Read the model definition and answer for the solid it produces. Units are mm, in the model's axes. Round coordinates to 2 decimals unless told otherwise and drop trailing zeros. Order: outer loops, then holes, each group sorted by start corner. A loop starts at its lowest first (then second) coordinate and runs counter-clockwise, first axis right, second up. Notation, with made-up numbers: (34, 37.5) -> (80, 37.5) arc R6 cw to (80, 43.5) -> close; hole circle Ø7 at (-23, 26.25). An arc over 180 degrees is marked (long way). Answer as a JSON object with one key per item and string values. Group by question number.
Item 1: Section A-A, the plane z = -97 is taken. Write down the section's boundary in (x, y), plus the area to 3 significant figures.
Item 2: Consider probe 1 along Z at (x, y) = (37.5, 192); probe 2 along Z at (x, y) = (107, 77); probe 3 along Y at (x, z) = (52, -43). Determine where each line is inside the solid, lowest interval first. Write a range as from..to.
Item 3: Given P1, Ø10, axis at x = 96, z = -154, coming from the -Y side; P2, Ø10, axis at x = 42.5, y = 77.5, coming from the -Z side; P3, Ø3, axis at x = 44, y = 302, coming from the +Z side, each flat-ended and moving along its own axis, determine where each tip first touches the part or whether it passes through.
Item 4: The mould has two halves that part along Z. Classify faces 1 (the flat face through (0, 343, 91)), 2 (the flat face through (78.88, 322.594, -38.801)), 3 (the flat face through (78.88, 352.375, -44.693)): pulls with the +Z half, pulls with the -Z half, needs draft (parallel to the pull), parting line crosses it, or undercut.
Autodesk Inventor part; units mm, degrees
ref_plane "YZ Plane" through (0, 0, 0) normal (1, 0, 0) x (0, 1, 0)
ref_plane "XY Plane" through (0, 0, 0) normal (0, 0, 1) x (1, 0, 0)
sketch "Sketch2" plane through (0, 0, 0) normal (1, 0, 0) x (0, 1, 0)
  line L0 (0, 380) -> (0, 410)
  line L1 (0, -230) -> (0, -200)
  line L2 (0, 0) -> (0, 132.8644)
  line L3 (295.6158, -112.924) -> (350.339, 37.4268)
  line L4 (379.3536, 29.4296) -> (324.6304, -120.9212)
  ellipse E0 centre (0, 0) end of major axis (358.1699, 0) minor radius 200 (0, -200) -> (295.6158, -112.924) ccw
  ellipse E1 centre (0, 0) end of major axis (352.0508, 0) minor radius 380 (350.339, 37.4268) -> (0, 380) ccw
  ellipse E2 centre (0, 0) end of major axis (381.6296, 0) minor radius 230 (0, -230) -> (324.6304, -120.9212) ccw
  ellipse E3 centre (0, 0) end of major axis (380.3347, 0) minor radius 410 (379.3536, 29.4296) -> (0, 410) ccw
  point P0 (0, 0)
  dimension "d10" = 30
  dimension "d11" = 30
  dimension "d12" = 0
  dimension "d16" = 380
  dimension "d17" = 200
  dimension "d25" = 20
  dimension "d26" = 160
  dimension "d27" = 30
  dimension "d28" = 160
extrude "Extrusion1" add sketch "Sketch2" along normal blind 160
sketch "Sketch3" plane through (0, 0, 0) normal (-1, 0, 0) x (0, 0, 1)
  line L0 (171.5389, -307.9404) -> (-54.4979, 313.0907)
  line L1 (-120.9212, 324.6304) -> (29.4296, 379.3536)
  line L2 (-111.428, -307.9404) -> (360.7046, -307.9404)
  line L3 (76.7879, 236.8347) -> (76.7879, -307.9404)
  point P0 (0, 0)
  dimension "d31" = 94.751
sketch "Sketch4" plane through (0, 0, 380) normal (0, -1, 0) x (1, 0, 0)
  line L0 (160, 30) -> (160, 0)
  line L1 (160, -610) -> (160, -500.9212)
  line L2 (160, 30) -> (160, -610)
  line L3 (160, 0) -> (160, -342.5732)
  ellipse E0 centre (160, -290) end of major axis (390, -290) minor radius 320 (160, -610) -> (160, 30) ccw
  line L4 (0, 30) -> (160, 30)
  line L5 (0, 0) -> (160, 0)
  ellipse E1 centre (160, -290) end of major axis (360, -290) minor radius 290 (160, -580) -> (160, 0) ccw
  point P0 (0, -380)
  dimension "d33" = 200
  dimension "d34" = 230
  dimension "d32" = 320
ref_plane "Work Plane3" through (0, 0, 90) normal (0, 0, -1) x (-1, 0, 0)
ref_plane "Work Plane1" through (0, 0, -230) normal (0, 0, -1) x (-1, 0, 0)
ref_plane "Work Plane2" through (0, 0, 410) normal (0, 0, 1) x (1, 0, 0)
sketch "Sketch6" plane through (0, 0, 90) normal (0, 0, -1) x (-1, 0, 0)
  line L0 (-160, 371.0583) -> (0, 371.0583)
  line L1 (0, 371.0583) -> (0, 342.0343)
  line L2 (0, 342.0343) -> (-160, 342.0343)
  line L3 (-160, 342.0343) -> (-160, 371.0583)
  ellipse E0 centre (-160, -10) end of major axis (-390, -10) minor radius 381.0583 (-160, 371.0583) -> (-390, -10) ccw
  line L4 (-160, 0) -> (-160, 350.339)
  line L5 (-160, 342.0343) -> (-160, 371.0583)
  line L6 (-360, -10) -> (-390, -10)
  ellipse E1 centre (-160, -10) end of major axis (-360, -10) minor radius 352.0343 (-160, 342.0343) -> (-360, -10) ccw
  ellipse E2 centre (-160, -10) end of major axis (-403.0676, -10) minor radius 410.7244 (-34.7861, 342.0343) -> (-69.2995, 371.0583) ccw
  line L7 (0, 0) -> (-160, 0)
  point P0 (-160, 324.6304)
  dimension "d62" = 200
  dimension "d63" = 230
  dimension "d58" = 30
  dimension "d59" = 0
  dimension "d60" = 10
  dimension "d61" = 0
sketch "Sketch7" plane through (0, 0, 90) normal (0, 0, -1) x (-1, 0, 0)
  line L0 (0, 0) -> (-160, 0)
  ellipse E0 centre (-160, 0) end of major axis (-160, 365) minor radius 215 (-160, 365) -> (-375, 0) ccw
  line L1 (-160, 0) -> (-160, 350.339)
  line L2 (-375, 0) -> (-160, 0)
  line L3 (-160, 0) -> (-160, 365)
  line L4 (-160, 324.6304) -> (-160, 379.3536)
  dimension "d40" = 215
  dimension "d41" = 365
ref_plane "Work Plane4" through (210, 0, 0) normal (1, 0, 0) x (0, 0, -1)
sketch "Sketch10" plane through (160, 0, 0) normal (1, 0, 0) x (0, 0, -1)
  line L0 (120.9212, 324.6304) -> (-29.4296, 379.3536)
  ellipse E0 centre (0, 0) end of major axis (-410, 0) minor radius 380.3347 (-29.4296, 379.3536) -> (-410, 0) ccw
  line L1 (-410, 0) -> (-380, 0)
  ellipse E1 centre (0, 0) end of major axis (-380, 0) minor radius 352.0508 (-37.4268, 350.339) -> (-380, 0) ccw
  line L2 (-37.4268, 350.339) -> (112.924, 295.6158)
  ellipse E2 centre (0, 0) end of major axis (0, -358.1699) minor radius 200 (200, 0) -> (112.924, 295.6158) ccw
  line L3 (200, 0) -> (230, 0)
  ellipse E3 centre (0, 0) end of major axis (0, 381.6296) minor radius 230 (230, 0) -> (120.9212, 324.6304) ccw
  point P0 (0, 0)
ref_plane "Work Plane5" through (0, -10, 0) normal (0, 1, 0) x (-1, 0, 0)
sketch "Sketch11" plane through (0, -10, 0) normal (0, 1, 0) x (-1, 0, 0)
  line L0 (-160, -200) -> (-160, -230)
  ellipse E0 centre (-160, 90) end of major axis (-160, -230) minor radius 230 (-160, 410) -> (-160, -230) ccw
  line L1 (-160, -200) -> (-160, -112.924)
  ellipse E1 centre (-160, 90) end of major axis (-160, -200) minor radius 200 (-160, 380) -> (-160, -200) ccw
  line L2 (0, -230) -> (-160, -230)
  line L3 (-160, -200) -> (-160, -230)
  line L4 (0, 380) -> (-160, 380)
  line L5 (-160, 410) -> (-160, 380)
  line L6 (-160, 380) -> (-160, 410)
  point P0 (0, 0)
  dimension "d48" = 230
  dimension "d49" = 200
equation "\"d28\" = d26"
properties part number "eggshell_3dprintcore"
Values found:
{
 "1": {"outline": "(0, 301.41) -> (160, 301.41) -> (160, 333.34) -> (0, 333.34) -> close", "area": "5,110 mm2"},
 "2": {"probe 1": "-198.77..-168.84, 318.51..353.92", "probe 2": "-225.27..-195.32, 370.8..401.51", "probe 3": "321.07..352.99"},
 "3": {"P1": "y = 217.27", "P2": "z = -225.81", "P3": "z = 251.32"},
 "4": {"face 1": "needs draft", "face 2": "undercut", "face 3": "pulls with the -Z half"}
}
